Input: part model. Units: mm. Frame: model coordinates. A direction names the side the tool comes from. Give positions to 0.01 mm unless a question says otherwise; leave off trailing zeros. Loops run counter-clockwise (first coordinate to the right, second up) from the corner with the lowest first, then second, coordinate; pieces in that order, holes last. Notation, with made-up numbers: (58, -38.5) -> (88, -38.5) arc R33 ccw to (88, -6.5) -> close; hole circle Ø6 at (70.25, 42.25). An arc over 180 degrees is marked (long way). One line per question, with ' | ' between items.
from build123d import *

# Parameters (mm, degrees)
F_0120_CYLINDER_SKETCH_R    = 3.25
F_0120_CYLINDER_DEPTH       = 2.5
F_0121_FILLET_R             = 0.625
F_0122_EXTRUDE_DEPTH        = 1.385
F_0122_EXTRUDE_ROTATE_ANGLE = 120
F_0125_CYLINDER_SKETCH_R    = 1.2
F_0125_CYLINDER_DEPTH       = 49.7
F_0126_CONE_ROTATE_ANGLE    = 90


with BuildPart() as part:
    # 0120_cylinder_Sketch → 0120_cylinder (new body)
    with BuildSketch(Plane.XY):
        Circle(F_0120_CYLINDER_SKETCH_R)
    extrude(amount=F_0120_CYLINDER_DEPTH)

    # 0121_fillet
    f_0121_fillet_edges = [part.edges().sort_by_distance(p)[0] for p in [
        (-3.25, 0, 2.5),
    ]]
    fillet(f_0121_fillet_edges, radius=F_0121_FILLET_R)


with BuildPart() as body_2:
    # 0122_extrude_Sketch → 0122_extrude (new body)
    with BuildSketch(Plane.XY):
        Polygon((0, 0), (1.154700538, 0), (1.732050808, 1), (1.154700538, 2), (0, 2), (-0.577350269, 1), align=None)
    extrude(amount=F_0122_EXTRUDE_DEPTH)


with BuildPart() as body_2_1:
    # 0122_extrude_Rotate: read off the stored shape, not the designer's step
    # 0122_extrude_Rotate: moved
    add(body_2.part.rotate(Axis((0, 0, 0), (0, 0, 1)), F_0122_EXTRUDE_ROTATE_ANGLE))


with BuildPart() as body_2_2:
    # 0122_extrude_Translate: moved
    add(body_2_1.part.moved(Location((1.154700538, 0, 1.125))))


with BuildPart() as part_1:
    add(part.part)

    # 0124_sub: cut body 2
    add(body_2_2.part, mode=Mode.SUBTRACT)


with BuildPart() as body_2_2_1:
    # 0125_cylinder_Sketch → 0125_cylinder (new body)
    with BuildSketch(Plane.XY):
        Circle(F_0125_CYLINDER_SKETCH_R)
    extrude(amount=F_0125_CYLINDER_DEPTH)


with BuildPart() as body_2_2_2:
    # 0125_cylinder_Translate: moved
    add(body_2_2_1.part.moved(Location((0, 0, -49.7))))


with BuildPart() as body_3:
    # 0126_cone_Sketch → 0126_cone (revolve)
    with BuildSketch(Plane.XY, mode=Mode.PRIVATE) as f_0126_cone_sk:
        Polygon((0, 0), (1.2, 0), (0.9, 0.3), (0, 0.3), align=None)
    revolve(f_0126_cone_sk.sketch.rotate(Axis((0, -100, 0), (0, 1, 0)), 90), axis=Axis((0, -100, 0), (0, 1, 0)))


with BuildPart() as body_3_1:
    # 0126_cone_Rotate: moved
    add(body_3.part.rotate(Axis((0, 0, 0), (1, 0, 0)), F_0126_CONE_ROTATE_ANGLE))


with BuildPart() as body_3_2:
    # 0126_cone_Translate: moved
    add(body_3_1.part.moved(Location((0, 0, -50))))


with BuildPart() as body_2_2_3:
    add(body_2_2_2.part)

    # 0128_add: union body 3
    add(body_3_2.part)


with BuildPart() as part_2:
    add(part_1.part)

    # 0129_add: union body 2 2
    add(body_2_2_3.part)


solid = part_2.part
1. Section query A-A (x = 0). Output: boundary loops of the cut face in (y, z) (3 decimals), then the cut area to 3 significant figures.
Determined:
outline: (-3.25, 0) -> (-1.2, 0) -> (-1.2, -49.7) -> (-0.9, -49.7) -> (-1.2, -50) -> (1.2, -50) -> (0.9, -49.7) -> (1.2, -49.7) -> (1.2, 0) -> (3.25, 0) -> (3.25, 1.875) arc R0.625 ccw to (2.625, 2.5) -> (1, 2.5) -> (1, 1.125) -> (-1, 1.125) -> (-1, 2.5) -> (-2.625, 2.5) arc R0.625 ccw to (-3.25, 1.875) -> close | area: 133 mm2
2. Ray query, line 1 along Z through (x, y) = (-1, -2.25); line 2 along Y through (x, z) = (0, -29.5); line 3 along Z through (x, y) = (0.25, 0.25) (3 decimals). Return the intervals inside material, ascending. Write a range as from..to.
Determined:
line 1: z = 0..2.5 | line 2: y = -1.2..1.2 | line 3: z = -50..1.125
3. Pull-direction query (Y, two-part tool) for faces 4 (the flat face through (0.87, 0.49, 1.8)), 5 (the flat face through (1, -1, 2.5)), 6 (the cylindrical face through (0.65, 1.01, -25.2)); classes: pulls with the +Y half, pulls with the -Y half, needs draft (parallel to the pull), parting line crosses it, or undercut.
Determined:
face 4: undercut | face 5: needs draft | face 6: parting line crosses it
4. Pin query (flat end, axial travel): P1, Ø3, axis at y = 2.5, z = -4.5, coming from the -X side; P2, Ø3, axis at y = 1.5, z = -12.5, coming from the +X side; P3, Ø1.5, axis at y = -0.5, z = -3, coming from the -X side. Return the tip coordinate at first contact, or that it passes through.
Determined:
P1: stops at x = -0.66 | P2: stops at x = 1.2 | P3: stops at x = -1.2
5. Reachability of faces 1 (the flat face through (0, -1, 2)), 2 (the flat face through (0, 0, -50)), 3 (the flat face through (1.4, 0, 0)) from +Z, -Z, +X, -X, +Y, -Y: full face, straight path, thin tool, end or side. Return the list, or none.
Determined:
face 1: +Z | face 2: -Z, +X, -X, +Y, -Y | face 3: -Z
6. Section query B-B (z = -28.5). Output: boundary loops of the cut face in (x, y), then the cut area to 3 significant figures.
Determined:
outline: circle Ø2.4 at (0, 0) | area: 4.52 mm2
